Read the model definition and answer for the solid it produces. Units are mm, in the model's axes. Face numbers are marked on the shaded views. A direction names the side the tool comes from. Give positions to 0.01 mm unless a question says otherwise; leave off trailing zeros. Loops run counter-clockwise (first coordinate to the right, second up) from the corner with the lowest first, then second, coordinate; pieces in that order, holes last.
(1) Each of these flat-tipped pins is pushed along its axis until it touches: P1, Ø3, axis at x = 6.5, y = 18, coming from the -Z side; P2, Ø4.5, axis at x = 33.65, y = 22.5, coming from the -Z side; P3, Ø3, axis at x = -33.65, y = 7.5, coming from the +Z side. Where does it stop, or does it pass through?
(2) Which of the six approach directions +Z, -Z, +X, -X, +Y, -Y give full straight-line access (tool end or side, diameter ignored) to the marked faces 1 and 2?
(3) Straight lines are drawn through the part: probe 1 along X at (y, z) = (22.5, -20); probe 2 along X at (y, z) = (29, -0.5); probe 3 along Y at (x, z) = (33.65, -25). For each, find the intervals that lie inside material, in ascending order.
(4) Find section A-A, the plane z = -11. Write down the section's boundary in (x, y).
(5) Find section C-C, the plane x = 3. Write down the section's boundary in (y, z).
(6) Determine the mould class of the marked faces 3, 4 and 5 for opening direction X: pulls with the +X half, pulls with the -X half, needs draft (parallel to the pull), parting line crosses it, or undercut.
(7) Find section B-B, the plane z = -4. Write down the section's boundary in (x, y).
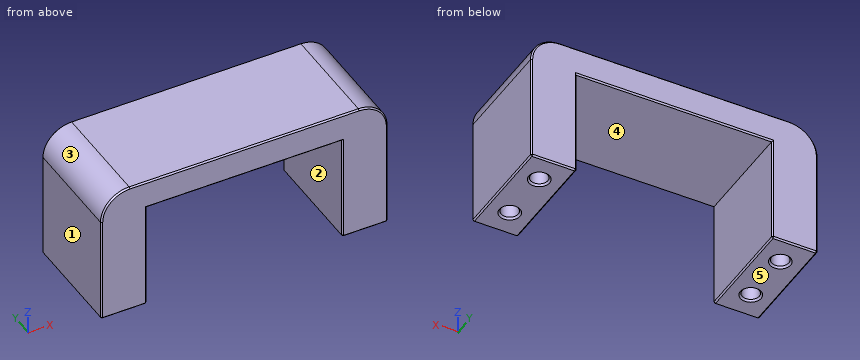
```python
from build123d import *

# Parameters (mm, degrees)
BOSS_EXTRUDE1_DEPTH             = 30
F_2_5MM_DOWEL_HOLE1_D           = 4.8
F_2_5MM_DOWEL_HOLE1_DEPTH       = 20
F_2_5MM_DOWEL_HOLE1_CSINK_D     = 5.8
F_2_5MM_DOWEL_HOLE1_CSINK_ANGLE = 90
F_2_5MM_DOWEL_HOLE1_TIP         = 1.442065486
FILLET1_R                       = 8
CHAMFER1_SIZE                   = 0.4


with BuildPart() as part:
    # Sketch1 → Boss-Extrude1 (new body)
    with BuildSketch(Plane(origin=(0, 0, 0), x_dir=(1, 0, 0), z_dir=(0, 1, 0))):
        Polygon((-40, 30), (-40, -8), (40, -8), (40, 30), (27.3, 30), (27.3, 0), (-27.3, 0), (-27.3, 30), align=None)
    extrude(amount=BOSS_EXTRUDE1_DEPTH)

    # Ø2.5mm Dowel Hole1
    with Locations(Plane(origin=(0, 0, -30), x_dir=(-1, 0, 0), z_dir=(0, 0, -1))):
        with Locations((33.65, 7.5), (-33.65, 22.5), (-33.65, 7.5), (33.65, 22.5)):
            CounterSinkHole(F_2_5MM_DOWEL_HOLE1_D / 2, F_2_5MM_DOWEL_HOLE1_CSINK_D / 2, depth=F_2_5MM_DOWEL_HOLE1_DEPTH, counter_sink_angle=F_2_5MM_DOWEL_HOLE1_CSINK_ANGLE)
            with Locations((0, 0, -(F_2_5MM_DOWEL_HOLE1_DEPTH + F_2_5MM_DOWEL_HOLE1_TIP / 2))):  # 118° drill point
                Cone(0, F_2_5MM_DOWEL_HOLE1_D / 2, F_2_5MM_DOWEL_HOLE1_TIP, mode=Mode.SUBTRACT)

    # Fillet1
    fillet1_edges = [part.edges().sort_by_distance(p)[0] for p in [
        (40, 15, 8),
        (-40, 15, 8),
    ]]
    fillet(fillet1_edges, radius=FILLET1_R)

    # Chamfer1
    chamfer1_edges = [part.edges().sort_by_distance(p)[0] for p in [
        (-40, 0, -15),
        (-33.65, 0, -30),
        (-27.3, 15, -30),
        (27.3, 15, -30),
        (40, 15, -30),
        (-40, 15, -30),
        (33.65, 30, -30),
        (27.3, 30, -15),
        (0, 30, 0),
        (-27.3, 30, -15),
        (0, 0, 8),
        (0, 30, 8),
        (40, 0, -15),
        (37.656854249, 0, 5.656854249),
        (-37.656854249, 0, 5.656854249),
        (40, 30, -15),
        (37.656854249, 30, 5.656854249),
        (-33.65, 30, -30),
        (-37.656854249, 30, 5.656854249),
        (-27.3, 0, -15),
        (-40, 30, -15),
        (0, 0, 0),
        (27.3, 0, -15),
        (33.65, 0, -30),
    ]]
    chamfer(chamfer1_edges, length=CHAMFER1_SIZE)


solid = part.part
```
Entries:
1. P1: stops at z = 0
1. P2: stops at z = -9.91
1. P3: stops at z = 8
2. face 1: +Z, -Z, -X, +Y, -Y
2. face 2: -Z, +Y, -Y
3. probe 1: x = -40 to -36.05, -31.25 to -27.3, 27.3 to 31.25, 36.05 to 40
3. probe 2: x = -40 to -27.3, 27.3 to 40
3. probe 3: y = 0 to 5.1, 9.9 to 20.1, 24.9 to 30
4. outline: (-40, 0.4) - (-39.6, 0) - (-27.7, 0) - (-27.3, 0.4) - (-27.3, 29.6) - (-27.7, 30) - (-39.6, 30) - (-40, 29.6) - close; (27.3, 0.4) - (27.7, 0) - (39.6, 0) - (40, 0.4) - (40, 29.6) - (39.6, 30) - (27.7, 30) - (27.3, 29.6) - close; hole circle Ø4.8 at (-33.65, 7.5); hole circle Ø4.8 at (-33.65, 22.5); hole circle Ø4.8 at (33.65, 7.5); hole circle Ø4.8 at (33.65, 22.5)
5. outline: (0, 0.4) - (0.4, 0) - (29.6, 0) - (30, 0.4) - (30, 7.6) - (29.6, 8) - (0.4, 8) - (0, 7.6) - close
6. face 3: pulls with the -X half
6. face 4: undercut
6. face 5: needs draft
7. outline: (-40, 0.4) - (-39.6, 0) - (-27.7, 0) - (-27.3, 0.4) - (-27.3, 29.6) - (-27.7, 30) - (-39.6, 30) - (-40, 29.6) - close; (27.3, 0.4) - (27.7, 0) - (39.6, 0) - (40, 0.4) - (40, 29.6) - (39.6, 30) - (27.7, 30) - (27.3, 29.6) - close
